Here's how the part is built. I have some questions about the finished solid (model axes, mm). Face numbers are marked on the shaded views. A direction names the side the tool comes from. Round coordinates to 2 decimals unless told otherwise and drop trailing zeros. Loops run counter-clockwise (first coordinate to the right, second up) from the corner with the lowest first, then second, coordinate; pieces in that order, holes last. Notation, with made-up numbers: M 75,3.5 L 113,3.5 A13 ccw 113,7.5 Z; hole C 11.5,-36.75 d5. An arc over 180 degrees is marked long. Answer as a JSON object with one key per item and string values.
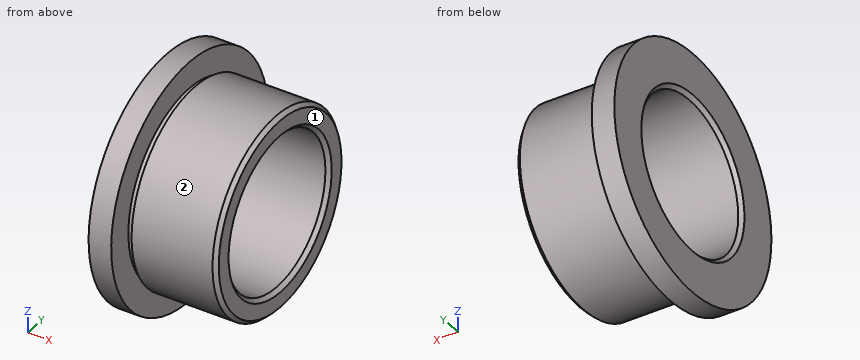
from build123d import *

# Parameters (mm, degrees)
ZKOSIT1_SIZE = 0.5


with BuildPart() as part:
    # Skica1 → Otočit kolem osy1 (revolve)
    with BuildSketch(Plane.XY, mode=Mode.PRIVATE) as oto_it_kolem_osy1_sk:
        Polygon((0, 16), (0, 10), (15, 10), (15, 13), (3.75, 13), (3.75, 12.5), (3, 12.5), (3, 16), align=None)
    revolve(oto_it_kolem_osy1_sk.sketch.rotate(Axis((0, 0, 0), (1, 0, 0)), 90), axis=Axis((0, 0, 0), (1, 0, 0)))

    # Zkosit1
    zkosit1_edges = [part.edges().sort_by_distance(p)[0] for p in [
        (0, 0, -10),
        (15, 0, -10),
        (15, 0, -13),
    ]]
    chamfer(zkosit1_edges, length=ZKOSIT1_SIZE)


solid = part.part
Item 1: On a 3-axis mill with a long thin cutter (end or side, diameter ignored), from which of +Z, -Z, +X, -X, +Y, -Y can I reach the whole of each face in a straight line? I mean the marked faces 1 and 2. Say none if no direction works.
Resolved:
{"face 1": "+Z, -Z, +X, +Y, -Y", "face 2": "+X"}
Item 2: I want a section at C-C, the plane x = 6.25. Please give me the cut outline in (y, z), then the cut area to 3 significant figures.
Resolved:
{"outline": "C 0,0 d26; hole C 0,0 d20", "area": "217 mm²"}
Item 3: I want a section at A-A, the plane y = 0. Please give me the cut outline in (x, z), then the cut area to 4 significant figures.
Resolved:
{"outline": "M 0,-16 L 3,-16 L 3,-12.5 L 3.75,-12.5 L 3.75,-13 L 14.5,-13 L 15,-12.5 L 15,-10.5 L 14.5,-10 L 0.5,-10 L 0,-10.5 Z; M 0,10.5 L 0.5,10 L 14.5,10 L 15,10.5 L 15,12.5 L 14.5,13 L 3.75,13 L 3.75,12.5 L 3,12.5 L 3,16 L 0,16 Z", "area": "106.5 mm²"}
Item 4: Please list where these lines run through material, in increasing order: probe 1 along Y at (x, z) = (8.5, 0); probe 2 along Z at (x, y) = (1, -0.5); probe 3 along Z at (x, y) = (6.5, 8). Write a range as from..to.
Resolved:
{"probe 1": "-13..-10, 10..13", "probe 2": "-15.99..-9.99, 9.99..15.99", "probe 3": "-10.25..-6, 6..10.25"}
Item 5: I'm going to push flat-ended pins straight in: pin 1 Ø1 at (x, z) = (9.5, 1.5) entering from +Y; pin 2 Ø1.5 at (x, y) = (3, 10) entering from +Z; pin 3 Ø5 at (x, z) = (6, 5) entering from +Y. Where does each tip first touch, or does it pass through?
Resolved:
{"pin 1": "y = 12.96", "pin 2": "z = 13.06", "pin 3": "y = 12.76"}
